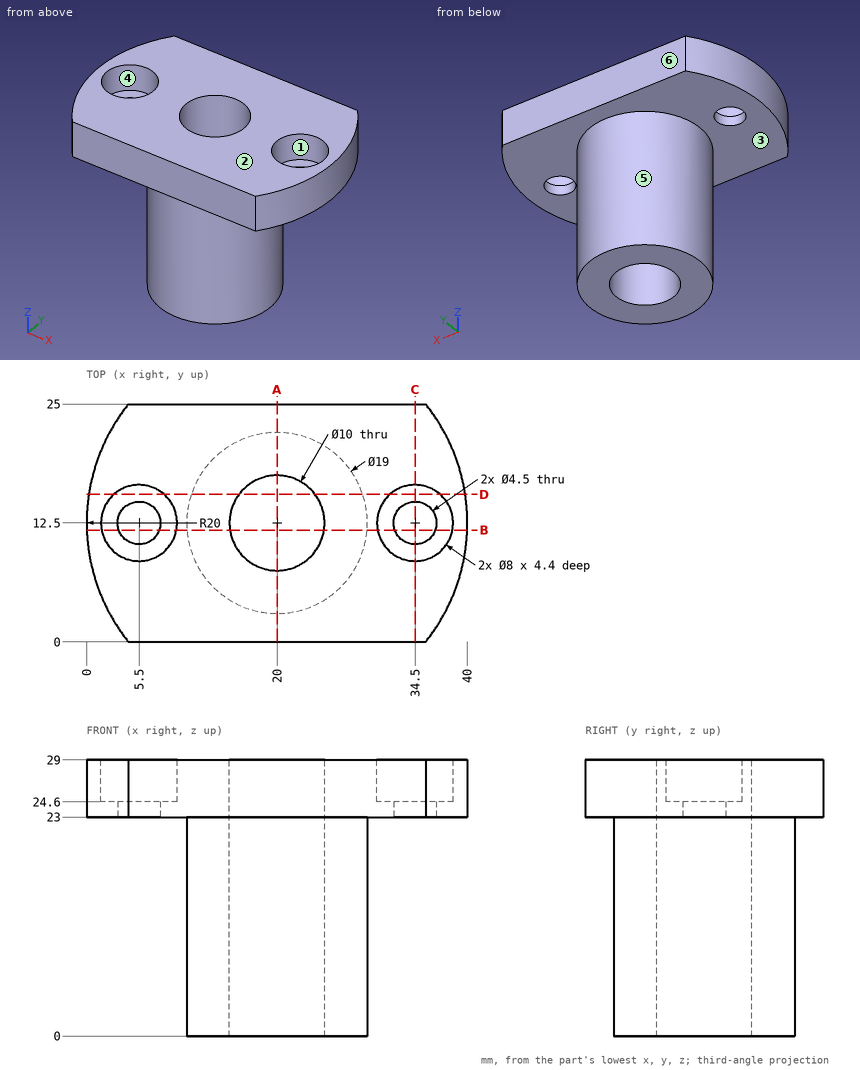
Geometry check sheet. Reference: drawing and pictorial views, mm from the part's lowest x, y, z. A direction names the side the tool comes from. Round coordinates to 2 decimals unless told otherwise and drop trailing zeros. Write each loop counter-clockwise with the first axis right and the second up, starting at its lowest first coordinate (ties: lowest second). Pieces come first, ordered by that corner, then holes.
(1) Section check B-B (y = 11.75). Enter the section's corners in (x, z).
Returned:
outline: (0.01, 23) - (3.38, 23) - (3.38, 24.6) - (1.57, 24.6) - (1.57, 29) - (0.01, 29) - close; (7.62, 23) - (10.53, 23) - (10.53, 0) - (15.06, 0) - (15.06, 29) - (9.43, 29) - (9.43, 24.6) - (7.62, 24.6) - close; (24.94, 0) - (29.47, 0) - (29.47, 23) - (32.38, 23) - (32.38, 24.6) - (30.57, 24.6) - (30.57, 29) - (24.94, 29) - close; (36.62, 23) - (39.99, 23) - (39.99, 29) - (38.43, 29) - (38.43, 24.6) - (36.62, 24.6) - close
(2) Mould release check, pull along Y, two halves, no side actions. Record for the marked faces 4, 5 and 6: pulls with the +Y half, pulls with the -Y half, needs draft (parallel to the pull), parting line crosses it, or undercut.
Returned:
face 4: undercut
face 5: parting line crosses it
face 6: pulls with the +Y half
(3) Section check A-A (x = 20). Enter the section's corners in (y, z), plus the area to 3 significant figures.
Returned:
outline: (0, 23) - (3, 23) - (3, 0) - (7.5, 0) - (7.5, 29) - (0, 29) - close; (17.5, 0) - (22, 0) - (22, 23) - (25, 23) - (25, 29) - (17.5, 29) - close
area: 297 mm2
(4) Depth check by flat-ended pin: pin 1 Ø5 at (x, y) = (34.5, 12.5) entering from +Z; pin 2 Ø2.5 at (x, y) = (34.5, 12.5) entering from -Z; pin 3 Ø3 at (y, z) = (3, 16) entering from +X; pin 4 Ø4 at (y, z) = (15, 25) entering from -X. Enter the tip coordinate at first touch or a pass-through.
Returned:
pin 1: stops at z = 24.6
pin 2: passes through
pin 3: stops at x = 25.12
pin 4: stops at x = 0.01
(5) Access from +Z, -Z, +X, -X, +Y, -Y to the whole of each face (thin tool, end or side, straight path). Record for the marked faces 1, 2 and 3.
Returned:
face 1: +Z
face 2: +Z, +X, -X, +Y, -Y
face 3: -Z
(6) Section check D-D (y = 15.5). Enter the section's corners in (x, z).
Returned:
outline: (0.23, 23) - (10.99, 23) - (10.99, 0) - (16, 0) - (16, 29) - (8.15, 29) - (8.15, 24.6) - (2.85, 24.6) - (2.85, 29) - (0.23, 29) - close; (24, 0) - (29.01, 0) - (29.01, 23) - (39.77, 23) - (39.77, 29) - (37.15, 29) - (37.15, 24.6) - (31.85, 24.6) - (31.85, 29) - (24, 29) - close
(7) Section check C-C (x = 34.5). Enter the section's corners in (y, z), plus the area to 3 significant figures.
Returned:
outline: (0, 23) - (10.25, 23) - (10.25, 24.6) - (8.5, 24.6) - (8.5, 29) - (0, 29) - close; (14.75, 23) - (25, 23) - (25, 29) - (16.5, 29) - (16.5, 24.6) - (14.75, 24.6) - close
area: 108 mm2
(8) Material ranges on line 1 (Y direction, x = 34.5, z = 26.65); line 2 (Y direction, x = 20, z = 11); line 3 (Z direction, x = 5, y = 7.25), recorded low to high.
Returned:
line 1: y = 0 to 8.5, 16.5 to 25
line 2: y = 3 to 7.5, 17.5 to 22
line 3: z = 23 to 29
